from build123d import *

# Parameters (mm, degrees)
F0_W     = 224.3
F0_H     = 68.4
F1_DEPTH = 5
F2_DEPTH = 3


with BuildPart() as f1:
    # F0 (on Top) → F1 (new body)
    with BuildSketch(Plane.XY):
        Polygon((124.15, -46.2), (124.15, 46.2), (10, 46.2), (-10, 46.2), (-124.15, 46.2), (-124.15, -46.2), align=None)
        Rectangle(F0_W, F0_H, mode=Mode.SUBTRACT)
    extrude(amount=F1_DEPTH)

    # F0 (on Top) → F2 (join)
    with BuildSketch(Plane.XY):
        with BuildLine():
            Line((-10, 46.2), (10, 46.2))
            Line((10, 46.2), (10, 51.2))
            ThreePointArc((10, 51.2), (12.928932, 58.271068), (20, 61.2))
            Line((20, 61.2), (80, 61.2))
            Line((80, 61.2), (80, 76.2))
            Line((80, 76.2), (10, 76.2))
            Line((10, 76.2), (0, 76.2))
            ThreePointArc((0, 76.2), (-7.071068, 73.271068), (-10, 66.2))
            Line((-10, 66.2), (-10, 46.2))
        make_face()
    extrude(amount=F2_DEPTH)


solid = f1.part
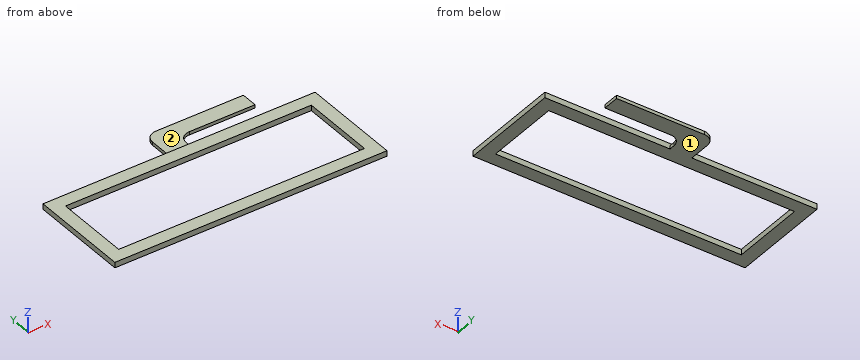
Design review of the part built by this model. Coordinates are the model's own, in mm. Face numbers are marked on the shaded views. A direction names the side the tool comes from. Give positions to 0.01 mm unless a question says otherwise; leave off trailing zeros. Loops run counter-clockwise (first coordinate to the right, second up) from the corner with the lowest first, then second, coordinate; pieces in that order, holes last. Notation, with made-up numbers: M -38.75,-28 L 15.25,-28 A26 ccw 15.25,-7 Z; hole C 81.25,-25.75 d8. An arc over 180 degrees is marked long. Answer as a JSON object with one key per item and string values.
Item 1: We need section D-D (x = -35.5). State the section outline as (y, z) points.
Output values:
{"outline": "M -46.2,0 L -34.2,0 L -34.2,5 L -46.2,5 Z; M 34.2,0 L 46.2,0 L 46.2,5 L 34.2,5 Z"}
Item 2: We need section C-C (z = 3.8). State the section outline as (x, y) points, and give its area (3 significant figures).
Output values:
{"outline": "M -124.15,-46.2 L 124.15,-46.2 L 124.15,46.2 L -124.15,46.2 Z; hole M -112.15,-34.2 L 112.15,-34.2 L 112.15,34.2 L -112.15,34.2 Z", "area": "7,600 mm2"}
Item 3: We need section B-B (y = 7). State the section outline as (x, z) points.
Output values:
{"outline": "M -124.15,0 L -112.15,0 L -112.15,5 L -124.15,5 Z; M 112.15,0 L 124.15,0 L 124.15,5 L 112.15,5 Z"}
Item 4: Wall thickness on line 1 along Y through (x, z) = (30.5, 1.7); line 2 along Y through (x, z) = (94, 2.35); line 3 along X through (y, z) = (-6, 1.55): over which ranges is each line inside the solid? List them lowest first.
Output values:
{"line 1": "y = -46.2 to -34.2, 34.2 to 46.2, 61.2 to 76.2", "line 2": "y = -46.2 to -34.2, 34.2 to 46.2", "line 3": "x = -124.15 to -112.15, 112.15 to 124.15"}
Item 5: We need section A-A (x = 73). State the section outline as (y, z) points, and give its area (3 significant figures).
Output values:
{"outline": "M -46.2,0 L -34.2,0 L -34.2,5 L -46.2,5 Z; M 34.2,0 L 46.2,0 L 46.2,5 L 34.2,5 Z; M 61.2,0 L 76.2,0 L 76.2,3 L 61.2,3 Z", "area": "165 mm2"}
Item 6: Machinability: for the marked faces 1 and 2, which of the approach directions +Z, -Z, +X, -X, +Y, -Y give a long, thin tool a straight path to every point of the face, cutting with its end or side? Answer none if there is none.
Output values:
{"face 1": "-Z, +X, -X, +Y, -Y", "face 2": "+Z, +X, -X, +Y"}
Item 7: For P1, Ø2.5, axis at y = 49.5, z = 1, coming from the +X side; P2, Ø2.5, axis at y = 53.5, z = 1, coming from the -X side, all flat-tipped, find the tip position at first contact; note any pin that passes through.
Output values:
{"P1": "stops at x = 10", "P2": "stops at x = -10"}
